```python
from build123d import *

# Parameters (mm, degrees)
SKETCH4_R               = 4
BOSS_EXTRUDE6_DEPTH     = 13
CUT_EXTRUDE3_DEPTH      = 1
CUT_EXTRUDE3_DEPTH_BACK = 11
SKETCH6_R               = 1.5
CUT_EXTRUDE4_DEPTH      = 3
BOSS_EXTRUDE7_DEPTH     = 67
SKETCH8_R               = 6
BOSS_EXTRUDE8_DEPTH     = 3


with BuildPart() as part:
    # Sketch4 → Boss-Extrude6 (new body)
    with BuildSketch(Plane(origin=(0, 0, 0), x_dir=(1, 0, 0), z_dir=(0, 1, 0))):
        Circle(SKETCH4_R)
    extrude(amount=BOSS_EXTRUDE6_DEPTH)

    # Sketch5 → Cut-Extrude3 (cut, two sides)
    with BuildSketch(Plane.XZ) as cut_extrude3_sk:
        with BuildLine():
            Line((-3.708099244, -1.5), (-3.708099244, 1.5))
            ThreePointArc((-3.708099244, 1.5), (-4, 0), (-3.708099244, -1.5))
        make_face()
        with BuildLine():
            Line((3.708099244, -1.5), (3.708099244, 1.5))
            ThreePointArc((3.708099244, 1.5), (4, 0), (3.708099244, -1.5))
        make_face()
    extrude(amount=CUT_EXTRUDE3_DEPTH, mode=Mode.SUBTRACT)
    extrude(cut_extrude3_sk.sketch, amount=-CUT_EXTRUDE3_DEPTH_BACK, mode=Mode.SUBTRACT)

    # Sketch6 → Cut-Extrude4 (cut)
    with BuildSketch(Plane.ZY.offset(3.708099244)):
        with Locations((0, 5)):
            Circle(SKETCH6_R)
    extrude(amount=-CUT_EXTRUDE4_DEPTH, mode=Mode.SUBTRACT)

    # Sketch7 → Boss-Extrude7 (add)
    with BuildSketch(Plane(origin=(0, 13, 0), x_dir=(1, 0, 0), z_dir=(0, 1, 0))):
        with BuildLine():
            Line((1.5, 1.5), (1.5, 3.708099244))
            ThreePointArc((1.5, 3.708099244), (0, 4), (-1.5, 3.708099244))
            Line((-1.5, 3.708099244), (-1.5, 1.5))
            Line((-1.5, 1.5), (-3.708099244, 1.5))
            ThreePointArc((-3.708099244, 1.5), (-4, 0), (-3.708099244, -1.5))
            Line((-3.708099244, -1.5), (-1.5, -1.5))
            Line((-1.5, -1.5), (-1.5, -3.708099244))
            ThreePointArc((-1.5, -3.708099244), (0, -4), (1.5, -3.708099244))
            Line((1.5, -3.708099244), (1.5, -1.5))
            Line((1.5, -1.5), (3.708099244, -1.5))
            ThreePointArc((3.708099244, -1.5), (4, 0), (3.708099244, 1.5))
            Line((3.708099244, 1.5), (1.5, 1.5))
        make_face()
    extrude(amount=BOSS_EXTRUDE7_DEPTH)

    # Sketch8 → Boss-Extrude8 (add)
    with BuildSketch(Plane(origin=(0, 80, 0), x_dir=(1, 0, 0), z_dir=(0, 1, 0))):
        Circle(SKETCH8_R)
    extrude(amount=BOSS_EXTRUDE8_DEPTH)


solid = part.part
```
Build history of the part. All positions in model axes, mm. A direction names the side the tool comes from. Coordinates: 2 decimals unless noted, no trailing zeros. Order: outer loops, then holes, each group sorted by start corner. A loop starts at its lowest first (then second) coordinate and runs counter-clockwise, first axis right, second up. Notation, with made-up numbers: M 89,72 L 139,72 A16 ccw 139,80 Z; hole C 69,-8.75 d5. An arc over 180 degrees is marked long. One line per question, with ' | ' between items. Start each with the question number.
1. Cut at B-B (x = 0). Write the cut outline in (y, z).
2. Cut at A-A (y = 18.5). Write the cut outline in (x, z), plus the area to 4 significant figures.
3. Flat gauge pins, fed straight in: P1, Ø5, axis at x = 1.5, y = 24.5, coming from the +Z side; P2, Ø2.5, axis at x = 3, y = 32.5, coming from the +Z side; P3, Ø6, axis at y = 24.5, z = 4, coming from the +X side. Where does each tip first touch, or does it go through?
4. Tool access for faces 4 (the face through (3.708, 5, 0)), 5 (the face through (-3, 46, -1.5)), 6 (the face through (-1.5, 46, 3)): list every direction of +Z, -Z, +X, -X, +Y, -Y with a clear straight run to the whole face (end or side of a thin tool).
5. Mould opens along Z. For faces 1 (the face through (0, 0, 0)), 2 (the face through (-0.708, 5, 0)), 3 (the face through (-6, 81, 0)) say: +Z half, -Z half, draft (parallel to the pull), parting line (faces both ways), or undercut.
6. Wall check: line 1 along Y through (x, z) = (-2.3, 0); line 2 along X through (y, z) = (78, 1.75); line 3 along Y through (x, z) = (0, -4.75). Give the ranges that are in metal, low to high. Write a range as [from, to].
The answers:
1) outline: M 0,-4 L 80,-4 L 80,-6 L 83,-6 L 83,6 L 80,6 L 80,4 L 0,4 Z
2) outline: M -3.71,-1.5 L -1.5,-1.5 L -1.5,-3.71 A4 ccw 1.5,-3.71 L 1.5,-1.5 L 3.71,-1.5 A4 ccw 3.71,1.5 L 1.5,1.5 L 1.5,3.71 A4 ccw -1.5,3.71 L -1.5,1.5 L -3.71,1.5 A4 ccw Z | area: 37.85 mm2
3) P1: stops at z = 4 | P2: stops at z = 1.5 | P3: stops at x = 3.87
4) face 4: +Z, -Z, +X, -Y | face 5: -Z, -X | face 6: +Z, -X
5) face 1: draft | face 2: undercut | face 3: parting line
6) line 1: y = [0, 3.5], [6.5, 83] | line 2: x = [-1.5, 1.5] | line 3: y = [80, 83]
